```python
from build123d import *

# Parameters (mm, degrees)
SKETCH18_W                  = 12.7
SKETCH18_H                  = 215.9
BOSS_EXTRUDE3_DEPTH         = 12.7
F_32_0_116_DIAMETER_HOLE7_D = 2.9464
SKETCH29_W                  = 6.35
SKETCH29_H                  = 12.7
BOSS_EXTRUDE4_DEPTH         = 6.35
SKETCH30_W                  = 6.35
SKETCH30_H                  = 7.112
BOSS_EXTRUDE5_DEPTH         = 6.35
SKETCH33_W                  = 12.7
SKETCH33_H                  = 12.7
CUT_EXTRUDE1_DEPTH          = 6.35


with BuildPart() as part:
    # Sketch18 → Boss-Extrude3 (new body)
    with BuildSketch(Plane(origin=(0, 0, 0), x_dir=(1, 0, 0), z_dir=(0, 1, 0))):
        with Locations((-6.35, 95.25)):
            Rectangle(SKETCH18_W, SKETCH18_H)
    extrude(amount=BOSS_EXTRUDE3_DEPTH)

    # #32 (0.116) Diameter Hole7 (through all)
    with Locations(Plane(origin=(0, 12.7, 0), x_dir=(1, 0, 0), z_dir=(0, 1, 0))):
        with Locations((-6.35, 196.85), (-6.35, 133.35), (-6.35, -6.35)):
            Hole(F_32_0_116_DIAMETER_HOLE7_D / 2)

    # Sketch29 → Boss-Extrude4 (add)
    with BuildSketch(Plane.ZY.offset(12.7)):
        with Locations((-155.575, 6.35)):
            Rectangle(SKETCH29_W, SKETCH29_H)
    boss_extrude4 = extrude(amount=BOSS_EXTRUDE4_DEPTH)

    # Sketch30 → Boss-Extrude5 (add)
    with BuildSketch(Plane.ZY.offset(12.7)):
        with Locations((-149.225, 3.556)):
            Rectangle(SKETCH30_W, SKETCH30_H)
    boss_extrude5 = extrude(amount=BOSS_EXTRUDE5_DEPTH)

    # Mirror2: Boss-Extrude4, Boss-Extrude5 across plane
    add(boss_extrude4.mirror(Plane.ZY.offset(6.35)))
    add(boss_extrude5.mirror(Plane.ZY.offset(6.35)))

    # Sketch33 → Cut-Extrude1 (cut)
    with BuildSketch(Plane.ZY.offset(19.05)):
        with Locations((-152.4, 6.35)):
            Rectangle(SKETCH33_W, SKETCH33_H)
    extrude(amount=-CUT_EXTRUDE1_DEPTH, mode=Mode.SUBTRACT)


solid = part.part
```
Build history of the part. All positions in model axes, mm. A direction names the side the tool comes from. Give positions to 0.01 mm unless a question says otherwise; leave off trailing zeros. Loops run counter-clockwise (first coordinate to the right, second up) from the corner with the lowest first, then second, coordinate; pieces in that order, holes last. Notation, with made-up numbers: (34.25, 88) - (93.25, 88) arc R22 cw to (93.25, 115) - close; hole circle Ø11 at (41.25, -31). An arc over 180 degrees is marked (long way). Use a Markdown table: item, result.
(1) Wall check: line 1 along Z through (x, y) = (-6.35, 3.75); line 2 along X through (y, z) = (7.25, -196.85); line 3 along X through (y, z) = (4, -29). Give the ranges that are in metal, low to high.
Taken from the geometry:
| item | result |
|---|---|
| line 1 | -203.2 to -198.32, -195.38 to -134.82, -131.88 to 4.88, 7.82 to 12.7 |
| line 2 | -12.7 to -7.82, -4.88 to 0 |
| line 3 | -12.7 to 0 |
(2) Which spindle directions (+Z, -Z, +X, -X, +Y, -Y) get a long thin tool onto all of the face, cutting with end or side? Do faces 1 (the face through (3, 10, -152.4)), 2 (the face through (3, 4, -146.05)), 3 (the face through (-8, 12.7, -97)), 4 (the face through (0, 6, -181)), 5 (the face through (-6, 6, 12.7)). Say none if no direction does.
Taken from the geometry:
| item | result |
|---|---|
| face 1 | +Z, +X, +Y |
| face 2 | +Z, +X, +Y, -Y |
| face 3 | +Z, -Z, +X, -X, +Y |
| face 4 | -Z, +X, +Y, -Y |
| face 5 | +Z, +X, -X, +Y, -Y |
(3) Band-saw the part on C-C (x = 4). Give the cut face in (y, z), and give its area (3 significant figures).
Taken from the geometry:
| item | result |
|---|---|
| outline | (0, -158.75) - (12.7, -158.75) - (12.7, -152.4) - (7.11, -152.4) - (7.11, -146.05) - (0, -146.05) - close |
| area | 126 mm2 |
(4) Band-saw the part on A-A (y = 4). Give the cut face in (x, z).
Taken from the geometry:
| item | result |
|---|---|
| outline | (-12.7, -203.2) - (0, -203.2) - (0, -158.75) - (6.35, -158.75) - (6.35, -146.05) - (0, -146.05) - (0, 12.7) - (-12.7, 12.7) - close; hole circle Ø2.95 at (-6.35, -196.85); hole circle Ø2.95 at (-6.35, -133.35); hole circle Ø2.95 at (-6.35, 6.35) |
(5) Drop flat-ended pins along their axis: pin 1 Ø3 at (x, y) = (4.5, 9) entering from +Z; pin 2 Ø5 at (x, y) = (4, 5.5) entering from +Z; pin 3 Ø1.9 at (x, y) = (2.5, 7.5) entering from -Z. Give the stop position or say it passes through.
Taken from the geometry:
| item | result |
|---|---|
| pin 1 | z = -152.4 |
| pin 2 | z = -146.05 |
| pin 3 | z = -158.75 |
(6) Band-saw the part on B-B (z = -149). Give the cut face in (x, y).
Taken from the geometry:
| item | result |
|---|---|
| outline | (-12.7, 0) - (6.35, 0) - (6.35, 7.11) - (0, 7.11) - (0, 12.7) - (-12.7, 12.7) - close |
(7) Band-saw the part on D-D (z = -40.5). Give the cut face in (x, y).
Taken from the geometry:
| item | result |
|---|---|
| outline | (-12.7, 0) - (0, 0) - (0, 12.7) - (-12.7, 12.7) - close |
